Study the drawing (mm; zero at the part's minimum x, y, z) and answer. A direction names the side the tool comes from. Coordinates: 2 decimals unless noted, no trailing zeros. Write each loop counter-clockwise with the first axis right and the second up, starting at its lowest first coordinate (ties: lowest second). Pieces come first, ordered by that corner, then holes. Notation, with made-up numbers: (-16, -5.5) -> (3, -5.5) arc R26 cw to (3, 29.5) -> close; hole circle Ø11 at (8, 12.5). An arc over 180 degrees is marked (long way). Write item = value, one per line. Start each with the question number.
1) Section C-C (y = 27) is taken. Determine the outline of the cut face in (x, z).
2) Section B-B (z = 23.5) is taken. Determine the outline of the cut face in (x, y), plus the area to 3 significant figures.
3) A tool of negligible diameter and unlimited length cuts with its end or side. For the marked faces 1, 2 and 3, from which of +Z, -Z, +X, -X, +Y, -Y can it reach the whole face along a straight path? Write none if from no direction.
4) Section A-A (x = 17) is taken. Determine the outline of the cut face in (y, z), plus the area to 3 significant figures.
5) Section D-D (x = 12) is taken. Determine the outline of the cut face in (y, z), plus the area to 3 significant figures.
6) Flat-ended cylindrical pins translate along their axes: pin 1 Ø1 at (x, y) = (12.5, 15.5) entering from +Z; pin 2 Ø11 at (y, z) = (24, 27) entering from -X; pin 3 Ø4 at (x, y) = (18.5, 32.5) entering from +Z. Find the tip coordinate at first contact, or state that the pin passes through.
7) Find the intervals of material crossed by line 1 along Z through (x, y) = (29.5, 29); line 2 along Z through (x, y) = (14, 25); line 3 along Y through (x, z) = (5.5, 27), in increasing order. Write a range as from..to.
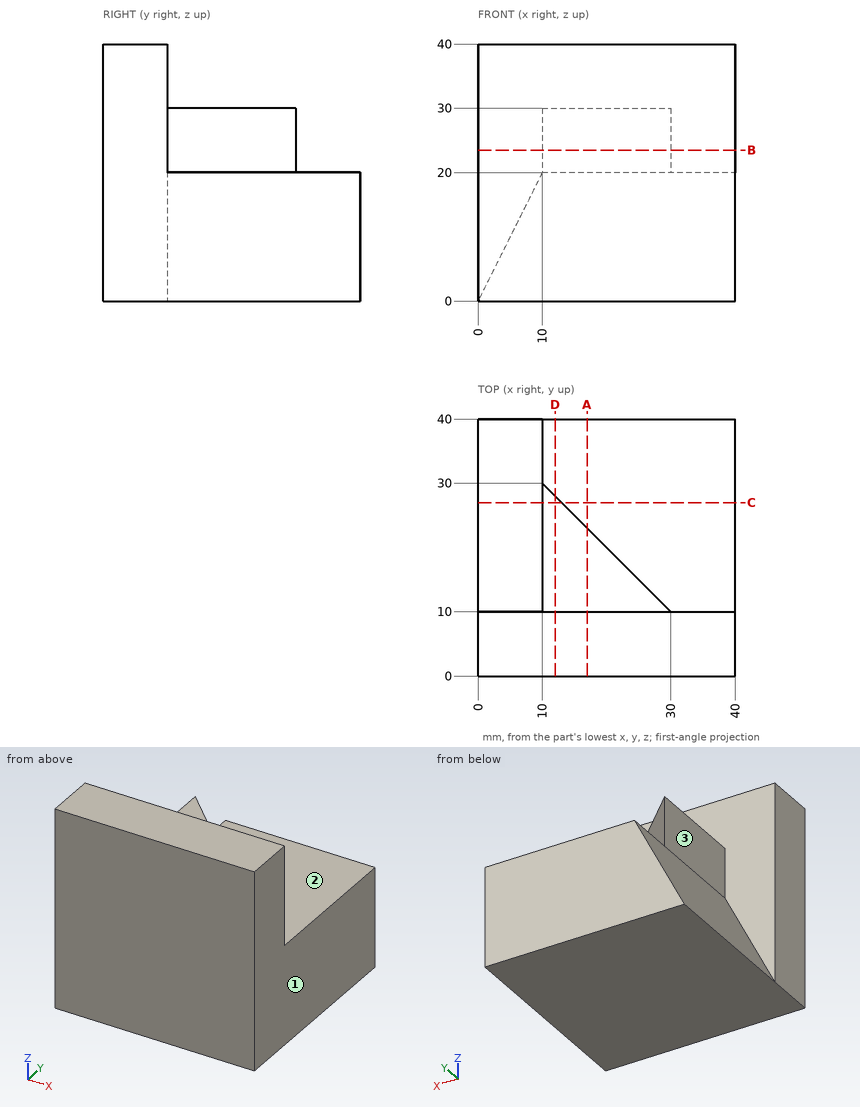
Answer key:
q1.outline = (0, 0) -> (40, 0) -> (40, 20) -> (13, 20) -> (13, 30) -> (10, 30) -> (10, 20) -> close
q2.outline = (0, 0) -> (40, 0) -> (40, 10) -> (30, 10) -> (10, 30) -> (10, 10) -> (0, 10) -> close
q2.area = 600 mm^2
q3.face_1 = +Z, -Z, +X, +Y, -Y
q3.face_2 = +Z, +X, +Y
q3.face_3 = +Z, -X, +Y
q4.outline = (0, 0) -> (40, 0) -> (40, 20) -> (23, 20) -> (23, 30) -> (10, 30) -> (10, 40) -> (0, 40) -> close
q4.area = 1,130 mm^2
q5.outline = (0, 0) -> (40, 0) -> (40, 20) -> (28, 20) -> (28, 30) -> (10, 30) -> (10, 40) -> (0, 40) -> close
q5.area = 1,180 mm^2
q6.pin_1 = 30
q6.pin_2 = 10
q6.pin_3 = 20
q7.line_1 = 0..20
q7.line_2 = 0..30
q7.line_3 = 0..10
